Autodesk Inventor part; units mm, degrees
ref_plane "YZ Plane" through (0, 0, 0) normal (1, 0, 0) x (0, 1, 0)
ref_plane "XZ Plane" through (0, 0, 0) normal (0, 1, 0) x (-1, 0, 0)
ref_plane "XY Plane" through (0, 0, 0) normal (0, 0, 1) x (1, 0, 0)
sketch "Sketch1" plane through (0, 0, 0) normal (0, 0, 1) x (1, 0, 0)
  line L0 (-11.7277, 11.2879) -> (33.7723, 11.2879)
  line L1 (33.7723, 11.2879) -> (33.7723, -42.7121)
  line L2 (33.7723, -42.7121) -> (-11.7277, -42.7121)
  line L3 (-11.7277, -42.7121) -> (-11.7277, 11.2879)
  line L4 (-11.7277, -9.7121) -> (-15.7277, -9.7121)
  line L5 (-15.7277, -9.7121) -> (-15.7277, -23.7121)
  line L6 (-15.7277, -23.7121) -> (-11.7277, -23.7121)
  line L7 (-11.7277, -23.7121) -> (-11.7277, -9.7121)
  line L8 (33.7723, -9.7121) -> (37.7723, -9.7121)
  line L9 (37.7723, -9.7121) -> (37.7723, -23.7121)
  line L10 (37.7723, -23.7121) -> (33.7723, -23.7121)
  line L11 (33.7723, -23.7121) -> (33.7723, -9.7121)
  point P0 (0, 0)
  dimension "d0" = 45.5
  dimension "d1" = 54
  dimension "d2" = 4
  dimension "d3" = 14
  dimension "d4" = 21
  dimension "d5" = 4
  dimension "d6" = 14
  dimension "d7" = 21
extrude "Extrusion1" add sketch "Sketch1" along normal blind 2 contours L0 L1 L2 L3
sketch "Sketch2" plane through (0, 0, 2) normal (0, 0, 1) x (1, 0, 0)
  line L0 (-11.7277, 11.2879) -> (-11.7277, -42.7121)
  line L1 (33.7723, -42.7121) -> (33.7723, 11.2879)
  line L2 (33.7723, 11.2879) -> (-11.7277, 11.2879)
  line L3 (-11.7277, -9.7121) -> (-15.7277, -9.7121)
  line L4 (-15.7277, -9.7121) -> (-15.7277, -25.7121)
  line L5 (-15.7277, -25.7121) -> (-11.7277, -25.7121)
  line L6 (-11.7277, -25.7121) -> (-11.7277, -9.7121)
  line L7 (33.7723, -9.7121) -> (37.7723, -9.7121)
  line L8 (37.7723, -9.7121) -> (37.7723, -25.7121)
  line L9 (37.7723, -25.7121) -> (33.7723, -25.7121)
  line L10 (33.7723, -25.7121) -> (33.7723, -9.7121)
  point P0 (0, 0)
  dimension "d10" = 4
  dimension "d11" = 16
  dimension "d12" = 21
  dimension "d13" = 4
extrude "Extrusion2" add sketch "Sketch2" against normal blind 7
sketch "Sketch3" plane through (33.7723, -9.7121, 2) normal (0, 1, 0) x (1, 0, 0)
  line L0 (4, 0) -> (4, 7)
  line L1 (0, 2) -> (0, 7)
  line L2 (0, 7) -> (0, 5.2)
  line L3 (0, 5.2) -> (2.1, 5.2)
  line L4 (2.1, 5.2) -> (0, 2)
  line L5 (0, 5.2) -> (0, 2)
  point P0 (-33.7723, 2)
  dimension "d16" = 1.8
  dimension "d17" = 2.1
extrude "Extrusion3" cut sketch "Sketch3" against normal blind 24.75
sketch "Sketch4" plane through (-15.7277, -9.7121, 2) normal (0, 1, 0) x (1, 0, 0)
  line L0 (4, 2) -> (4, 7)
  line L1 (4, 7) -> (4, 5.2)
  line L2 (4, 5.2) -> (1.9, 5.2)
  line L3 (1.9, 5.2) -> (4, 2)
  point P0 (15.7277, 2)
  dimension "d20" = 1.8
  dimension "d21" = 2.1
extrude "Extrusion4" cut sketch "Sketch4" against normal blind 176.5
sketch "Sketch5" plane through (-15.7277, -9.7121, 2) normal (0, 1, 0) x (1, 0, 0)
  line L0 (4, 5.2) -> (4, 7)
  line L1 (0, 7) -> (4, 7)
  line L2 (4, 2) -> (4, 0)
  line L3 (4, 2) -> (1.9, 5.2)
  line L4 (4, 5.2) -> (2.8188, 7)
  line L5 (4, 7) -> (4, 5.2)
  point P0 (15.7277, 2)
extrude "Extrusion5" cut sketch "Sketch5" against normal blind 3535.5
sketch "Sketch6" plane through (33.7723, -9.7121, 2) normal (0, 1, 0) x (1, 0, 0)
  line L0 (2.1, 5.2) -> (0, 2)
  line L1 (0, 7) -> (4, 7)
  line L2 (0, 5.2) -> (0, 7)
  line L3 (0, 5.2) -> (2.1, 5.2)
  line L4 (0, 5.2) -> (1.1813, 7)
  line L5 (0, 7) -> (0, 5.2)
  point P0 (-33.7723, 2)
extrude "Extrusion6" cut sketch "Sketch6" against normal blind 5309.5
properties part number "SkateBoxCover"
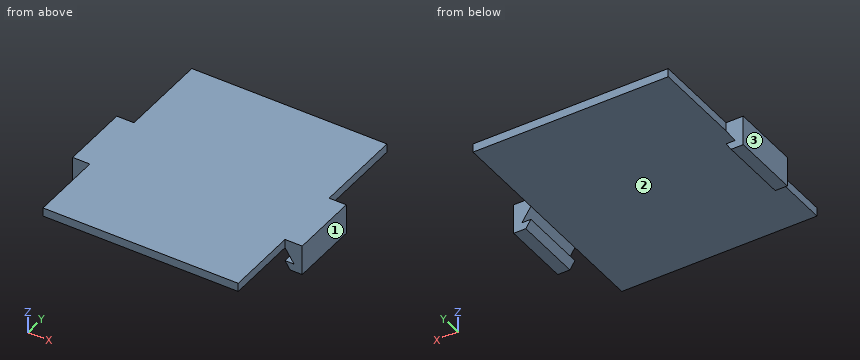
Check sheet for the modelled part. Datum: model origin and axes. Units: mm. Face numbers are marked on the shaded views. Round coordinates to 2 decimals unless told otherwise and drop trailing zeros. Write each loop counter-clockwise with the first axis right and the second up, starting at its lowest first coordinate (ties: lowest second). Pieces come first, ordered by that corner, then holes. Notation, with made-up numbers: (-14, 12) -> (3, 12) arc R31 cw to (3, 47) -> close; hole circle Ø5 at (76.5, 55.25). An arc over 180 degrees is marked (long way). Put each result on its own line as item: value.
(1) Sectioned sample at B-B (y = -19). Enter the section's corners in (x, z), plus the area to 3 significant figures.
Values found:
outline: (-15.73, -5) -> (-12.91, -5) -> (-11.73, -3.2) -> (-13.83, -3.2) -> (-11.73, 0) -> (33.77, 0) -> (35.87, -3.2) -> (33.77, -3.2) -> (34.95, -5) -> (37.77, -5) -> (37.77, 2) -> (-15.73, 2) -> close
area: 138 mm^2
(2) Material ranges on line 1 (Z direction, x = 31, y = -35); line 2 (X direction, y = -18, z = -0.25); line 3 (X direction, y = -21, z = -1.5), recorded low to high.
Values found:
line 1: z = 0 to 2
line 2: x = -15.73 to -11.89, 33.94 to 37.77
line 3: x = -15.73 to -12.71, 34.76 to 37.77
(3) Go/stop test with flat-tipped pins: pin 1 Ø1 at (y, z) = (-35, 1) entering from -X; pin 2 Ø2 at (x, z) = (-14.5, -2.5) entering from -Y; pin 3 Ø6 at (x, y) = (26, -16) entering from -Z; pin 4 Ø1 at (x, z) = (-4.5, -1) entering from -Y. Record where each tip stops, or that it passes through.
Values found:
pin 1: stops at x = -11.73
pin 2: stops at y = -25.71
pin 3: stops at z = 0
pin 4: passes through
(4) Sectioned sample at C-C (z = -4). Enter the section's corners in (x, y), plus the area to 3 significant figures.
Values found:
outline: (-15.73, -25.71) -> (-12.25, -25.71) -> (-12.25, -9.71) -> (-15.73, -9.71) -> close; (34.3, -25.71) -> (37.77, -25.71) -> (37.77, -9.71) -> (34.3, -9.71) -> close
area: 111 mm^2
(5) Mould release check, pull along X, two halves, no side actions. Record for the marked faces 1, 2 and 3: released by +X, released by -X, zero draft, split by the parting line, or undercut.
Values found:
face 1: released by +X
face 2: undercut
face 3: released by -X
(6) Sectioned sample at A-A (z = 0.75). Enter the section's corners in (x, y).
Values found:
outline: (-15.73, -25.71) -> (-11.73, -25.71) -> (-11.73, -42.71) -> (33.77, -42.71) -> (33.77, -25.71) -> (37.77, -25.71) -> (37.77, -9.71) -> (33.77, -9.71) -> (33.77, 11.29) -> (-11.73, 11.29) -> (-11.73, -9.71) -> (-15.73, -9.71) -> close
(7) Sectioned sample at D-D (x = 16). Enter the section's corners in (y, z), plus the area to 3 significant figures.
Values found:
outline: (-42.71, 0) -> (11.29, 0) -> (11.29, 2) -> (-42.71, 2) -> close
area: 108 mm^2
